Can you work these out from the model? Positions are in its coordinate system, mm. Round coordinates to 2 decimals unless told otherwise and drop trailing zeros. Loops run counter-clockwise (first coordinate to the right, second up) from the corner with the lowest first, then second, coordinate; pieces in that order, holes last.
(1) I want a section at A-A on z = -84. Write out the boundary of the cut face in (x, y), plus the area to 3 significant figures.
(2) If I drill on line 1 along X through (y, z) = (0.4, 84); line 2 along Z through (x, y) = (35, 0.6); line 3 along X through (y, z) = (0.3, -86), over which ranges is the centre line in solid material (lowest first)?
(3) I want a section at B-B on x = -37. Write out the boundary of the cut face in (y, z), plus the area to 3 significant figures.
(4) Thinking about a two-plate mould opening in X: for faces 1 (the face through (-35.5, 0.5, -86)), 2 (the face through (-1, 1, -1)), which applies, released by +X, released by -X, zero draft, split by the parting line, or undercut?
from build123d import *

# Parameters (mm, degrees)
SKETCH1_W               = 100
SKETCH1_H               = 200
BOSS_EXTRUDE1_DEPTH     = 1
SKETCH3_R               = 2.5
CUT_EXTRUDE1_DEPTH      = 112.807870922
MIRROR2_COPY_1_SKETCH_R = 2.5
MIRROR2_COPY_1_DEPTH    = 112.807870922


with BuildPart() as part:
    # Sketch1 → Boss-Extrude1 (new body)
    with BuildSketch(Plane(origin=(0, 0, 0), x_dir=(1, 0, 0), z_dir=(0, 1, 0))):
        Rectangle(SKETCH1_W, SKETCH1_H)
    extrude(amount=BOSS_EXTRUDE1_DEPTH)

    # Sketch3 → Cut-Extrude1 (cut, through all)
    with BuildSketch(Plane(origin=(0, 1, 0), x_dir=(1, 0, 0), z_dir=(0, 1, 0))):
        with Locations(Location((37, 84, 0), (0, 0, 270))):
            Circle(SKETCH3_R)
    cut_extrude1 = extrude(amount=-CUT_EXTRUDE1_DEPTH, mode=Mode.SUBTRACT)

    # Mirror1: Cut-Extrude1 across plane
    add(cut_extrude1.mirror(Plane(origin=(0, 0, 0), x_dir=(0, 0, 1), z_dir=(1, 0, 0))), mode=Mode.SUBTRACT)

    # Mirror2: Cut-Extrude1 across plane
    add(cut_extrude1.mirror(Plane.XY), mode=Mode.SUBTRACT)

    # Mirror2 copy 1 sketch → Mirror2 copy 1 (cut, through all)
    with BuildSketch(Plane(origin=(0, 1, 0), x_dir=(-1, 0, 0), z_dir=(0, 1, 0))):
        with Locations(Location((37, 84, 0), (0, 0, 270))):
            Circle(MIRROR2_COPY_1_SKETCH_R)
    extrude(amount=-MIRROR2_COPY_1_DEPTH, mode=Mode.SUBTRACT)


solid = part.part
Filled sheet:
1. outline: (-50, 0) - (-39.5, 0) - (-39.5, 1) - (-50, 1) - close; (-34.5, 0) - (34.5, 0) - (34.5, 1) - (-34.5, 1) - close; (39.5, 0) - (50, 0) - (50, 1) - (39.5, 1) - close
1. area: 90.0 mm2
2. line 1: x = -50 to -39.5, -34.5 to 34.5, 39.5 to 50
2. line 2: z = -100 to -85.5, -82.5 to 82.5, 85.5 to 100
2. line 3: x = -50 to -38.5, -35.5 to 35.5, 38.5 to 50
3. outline: (0, -100) - (1, -100) - (1, -86.5) - (0, -86.5) - close; (0, -81.5) - (1, -81.5) - (1, 81.5) - (0, 81.5) - close; (0, 86.5) - (1, 86.5) - (1, 100) - (0, 100) - close
3. area: 190 mm2
4. face 1: undercut
4. face 2: zero draft
